Geometry check sheet. Reference: the model listing, model coordinates, mm. Face numbers are marked on the shaded views. Round coordinates to 2 decimals unless told otherwise and drop trailing zeros. Order: outer loops, then holes, each group sorted by start corner. A loop starts at its lowest first (then second) coordinate and runs counter-clockwise, first axis right, second up. Notation, with made-up numbers: (57, -12) - (109, -12) arc R22 ccw to (109, 23) - close; hole circle Ø1 at (21, 74). An arc over 180 degrees is marked (long way). Return JSON: item names as keys, results as strings. Group by question number.
Q1. Draft check along Z on the marked faces 1, 2 and 3. Enter one of: pulls with the +Z half, pulls with the -Z half, needs draft (parallel to the pull), parting line crosses it, or undercut.
Q2. Sectioned sample at B-B, the plane y = -16.5. Give the number of separate pieces and of enclosed holes in the cut face, then the cut area to 3 significant figures.
Q3. Gauge pin test, flat ends, axial feed: pin 1 Ø3 at (y, z) = (-12, -11.5) entering from +X; pin 2 Ø21 at (x, z) = (0, 0) entering from +Y; pin 3 Ø8 at (x, y) = (-19, -14) entering from +Z; pin 4 Ø4 at (x, y) = (3.5, -18.5) entering from -Z. Record the tip position at first contact, or that the pin passes through.
Q4. Sectioned sample at D-D, the plane x = -21. Record the cut outline in (y, z), then the cut area to 3 significant figures.
Q5. Material ranges on line 1 along Z through (x, y) = (0, -5.25); line 2 along X through (y, z) = (-7.5, -3); line 3 along X through (y, z) = (-19, 4), recorded low to high.
Q6. Sectioned sample at C-C, the plane x = 0. Record the cut outline in (y, z).
Q7. Sectioned sample at A-A, the plane z = 0. Record the cut outline in (x, y).
```python
from build123d import *

# Parameters (mm, degrees)
F0_R     = 25
F0_R_2   = 3.5
F1_DEPTH = 25
F3_DEPTH = 25.001
F4_R     = 5
F5_R     = 13
F6_DEPTH = 25.001
F7_R     = 4.75
F8_DEPTH = 57.3563390593


with BuildPart() as f1:
    # F0 (on Front) → F1 (new body)
    with BuildSketch(Plane.XZ):
        Circle(F0_R)
        with Locations((0, -19)):
            Circle(F0_R_2, mode=Mode.SUBTRACT)
        with Locations((-19, 0)):
            Circle(F0_R_2, mode=Mode.SUBTRACT)
        with Locations((19, 0)):
            Circle(F0_R_2, mode=Mode.SUBTRACT)
        with Locations((0, 19)):
            Circle(F0_R_2, mode=Mode.SUBTRACT)
    extrude(amount=F1_DEPTH)

    # F2 (on Front) → F3 (cut, through all)
    with BuildSketch(Plane.XZ):
        with BuildLine():
            Line((-23.7634559673, 8.7634559673), (-16.2634559673, 8.7634559673))
            ThreePointArc((-16.2634559673, 8.7634559673), (-10.9601551084, 10.9601551084), (-8.7634559673, 16.2634559673))
            Line((-8.7634559673, 16.2634559673), (-8.7634559673, 23.7634559673))
            Line((-8.7634559673, 23.7634559673), (-23.7634559673, 23.7634559673))
            Line((-23.7634559673, 23.7634559673), (-23.7634559673, 8.7634559673))
        make_face()
        Polygon((1.4142135624, 29.6984848098), (29.6984848098, 1.4142135624), (61.3951798296, 33.6381491506), (33.3745288664, 61.6588001138), align=None)
        Polygon((-1.4142135624, -29.6984848098), (-29.6984848098, -1.4142135624), (-61.6588001138, -33.3745288664), (-33.6381491506, -61.3951798296), align=None)
        with BuildLine():
            ThreePointArc((16.2634559673, -8.7634559673), (10.9601551084, -10.9601551084), (8.7634559673, -16.2634559673))
            Line((8.7634559673, -16.2634559673), (8.7634559673, -23.7634559673))
            Line((8.7634559673, -23.7634559673), (23.7634559673, -23.7634559673))
            Line((23.7634559673, -23.7634559673), (23.7634559673, -8.7634559673))
            Line((23.7634559673, -8.7634559673), (16.2634559673, -8.7634559673))
        make_face()
    extrude(amount=F3_DEPTH, mode=Mode.SUBTRACT)

    # F4
    f4_edges = [f1.edges().sort_by_distance(p)[0] for p in [
        (-8.763456, -12.5, 23.413711),
        (-23.413711, -12.5, 8.763456),
        (8.763456, -12.5, -23.413711),
        (23.413711, -12.5, -8.763456),
        (23.952777, -12.5, 7.159921),
        (7.159921, -12.5, 23.952777),
        (-23.952777, -12.5, -7.159921),
        (-7.159921, -12.5, -23.952777),
    ]]
    fillet(f4_edges, radius=F4_R)

    # F5 (on Front) → F6 (cut, through all)
    with BuildSketch(Plane.XZ):
        Circle(F5_R)
    extrude(amount=F6_DEPTH, mode=Mode.SUBTRACT)

    # F7 (on face) → F8 (cut, through all)
    with BuildSketch(Plane(origin=(15.5563491861, 0, 15.5563491861), x_dir=(0.7071067812, 0, -0.7071067812), z_dir=(0.7071067812, 0, 0.7071067812))):
        with Locations((0, -12.5)):
            Circle(F7_R)
    extrude(amount=-F8_DEPTH, mode=Mode.SUBTRACT)


solid = f1.part
```
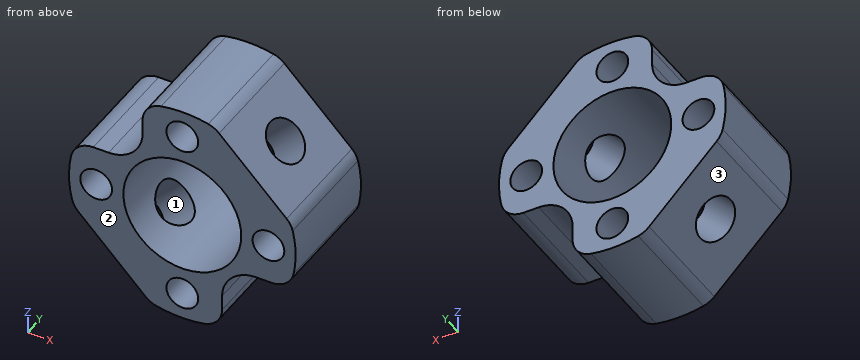
Reply:
{
 "1": {"face 1": "undercut", "face 2": "needs draft", "face 3": "pulls with the -Z half"},
 "2": {"separate pieces": "2", "enclosed holes": "4", "area": "824 mm^2"},
 "3": {"pin 1": "x = 12.14", "pin 2": "through", "pin 3": "z = 8.87", "pin 4": "z = -24.95"},
 "4": {"outline": "(-25, -10.11) - (0, -10.11) - (0, -2.87) - (-25, -2.87) - close; (-25, 2.87) - (0, 2.87) - (0, 8.58) - (-25, 8.58) - close", "area": "324 mm^2"},
 "5": {"line 1": "-25 to -22.5, -15.5 to -13, 13 to 15.5, 22.5 to 25", "line 2": "-24.82 to -20.8, -17.2 to -12.65, 12.65 to 17.2, 20.8 to 24.82", "line 3": "-24.68 to -12.37, 12.37 to 24.68"},
 "6": {"outline": "(-25, -25) - (0, -25) - (0, -22.5) - (-25, -22.5) - close; (-25, -15.5) - (0, -15.5) - (0, -13) - (-25, -13) - close; (-25, 13) - (0, 13) - (0, 15.5) - (-25, 15.5) - close; (-25, 22.5) - (0, 22.5) - (0, 25) - (-25, 25) - close"},
 "7": {"outline": "(-25, -25) - (-22.5, -25) - (-22.5, 0) - (-25, 0) - close; (-15.5, -25) - (-13, -25) - (-13, 0) - (-15.5, 0) - close; (13, -25) - (15.5, -25) - (15.5, 0) - (13, 0) - close; (22.5, -25) - (25, -25) - (25, 0) - (22.5, 0) - close"}
}
